from build123d import *

# Parameters (mm, degrees)
F1_DEPTH = 25.4
F3_DEPTH = 25.4
F4_DEPTH = 25.4


# Not quite as in the source:
# - a feature names something its author has since deleted; it is built from what else it names


with BuildPart() as f1:
    # F0 (on Top) → F1 (new body)
    with BuildSketch(Plane.XY):
        with BuildLine():
            ThreePointArc((128.3595710993, 553.8759422302), (1.1825358552, 549.8230168828), (-125.9080190212, 556.0210293531))
            Line((-125.9080190212, 556.0210293531), (-125.9080190212, -713.9789706469))
            ThreePointArc((-125.9080190212, -713.9789706469), (1.2643600135, -710.4779684085), (128.3595710993, -716.1240577698))
            Line((128.3595710993, -716.1240577698), (128.3595710993, 553.8759422302))
        make_face()
    extrude(amount=F1_DEPTH)

    # F2 (on face) → F3 (cut, through all)
    with BuildSketch(Plane.XY.offset(25.4)):
        with BuildLine():
            Line((21.1381499791, -78.9789706469), (0, -78.9789706469))
            Line((0, -78.9789706469), (0, -95.7576301918))
            ThreePointArc((0, -95.7576301918), (4.2283594629, -96.2864641581), (8.1962319091, -97.8403873742))
            Line((8.1962319091, -97.8403873742), (29.1618719602, -145.247048063))
            ThreePointArc((29.1618719602, -145.247048063), (59.1063769686, -142.7132397651), (62.4383196322, -112.8470092903))
            Line((62.4383196322, -112.8470092903), (27.7889794812, -88.7078500401))
            ThreePointArc((27.7889794812, -88.7078500401), (22.9597605864, -84.8714367544), (21.1381499791, -78.9789706469))
        make_face()
        with BuildLine():
            Line((0, -78.9789706469), (-21.1381499791, -78.9789706469))
            ThreePointArc((-21.1381499791, -78.9789706469), (-22.9597605864, -84.8714367544), (-27.7889794812, -88.7078500401))
            Line((-27.7889794812, -88.7078500401), (-62.4383196322, -112.8470092903))
            ThreePointArc((-62.4383196322, -112.8470092903), (-59.1063769686, -142.7132397651), (-29.1618719602, -145.247048063))
            Line((-29.1618719602, -145.247048063), (-8.3430390852, -97.9210786899))
            ThreePointArc((-8.3430390852, -97.9210786899), (-4.3094898358, -96.30729114), (0, -95.7576301918))
            Line((0, -95.7576301918), (0, -78.9789706469))
        make_face()
    extrude(amount=-F3_DEPTH, mode=Mode.SUBTRACT)

    # F2 (on face) → F4 (cut, through all)
    with BuildSketch(Plane.XY.offset(25.4)):
        with BuildLine():
            ThreePointArc((-27.7889794812, -69.2500912536), (-22.9597605864, -73.0865045393), (-21.1381499791, -78.9789706469))
            Line((-21.1381499791, -78.9789706469), (0, -78.9789706469))
            Line((0, -78.9789706469), (0, -62.2003111019))
            ThreePointArc((0, -62.2003111019), (-4.3094898358, -61.6506501538), (-8.3430390852, -60.0368626038))
            Line((-8.3430390852, -60.0368626038), (-29.1618719602, -12.7108932307))
            ThreePointArc((-29.1618719602, -12.7108932307), (-59.1063769686, -15.2447015287), (-62.4383196322, -45.1109320034))
            Line((-62.4383196322, -45.1109320034), (-27.7889794812, -69.2500912536))
        make_face()
        with BuildLine():
            Line((0, -62.2003111019), (0, -78.9789706469))
            Line((0, -78.9789706469), (21.1381499791, -78.9789706469))
            ThreePointArc((21.1381499791, -78.9789706469), (22.9597605864, -73.0865045393), (27.7889794812, -69.2500912536))
            Line((27.7889794812, -69.2500912536), (62.4383196322, -45.1109320034))
            ThreePointArc((62.4383196322, -45.1109320034), (59.1063769686, -15.2447015287), (29.1618719602, -12.7108932307))
            Line((29.1618719602, -12.7108932307), (8.1962319091, -60.1175539196))
            ThreePointArc((8.1962319091, -60.1175539196), (4.2283594629, -61.6714771356), (0, -62.2003111019))
        make_face()
    extrude(amount=-F4_DEPTH, mode=Mode.SUBTRACT)


solid = f1.part
Read the model definition and answer for the solid it produces. Units are mm, in the model's axes. A direction names the side the tool comes from. Round coordinates to 2 decimals unless told otherwise and drop trailing zeros. Order: outer loops, then holes, each group sorted by start corner. A loop starts at its lowest first (then second) coordinate and runs counter-clockwise, first axis right, second up. Notation, with made-up numbers: (41.5, -4) - (86.5, -4) arc R27 ccw to (86.5, 26) - close; hole circle Ø2 at (-29.5, 29.25). An arc over 180 degrees is marked (long way). Use one line per item in the form item = value. Start each with the question number.
(1) A flat-ended cylindrical pin translates along its axis: pin 1 Ø8 at (x, z) = (-59, 16) entering from +Y. Find the tip coordinate at first contact, or state that the pin passes through.
(2) Find the intervals of material crossed by line 1 along Y through (x, z) = (33.5, 14.25); line 2 along Y through (x, z) = (32, 1.25); line 3 along Y through (x, z) = (12, 10), in increasing order. Write a range as from..to.
(3) For faces 4 (the face through (-29, -71, 0)), 5 (the face through (44.87, -57.35, 12.88)), determine the directions among +Z, -Z, +X, -X, +Y, -Y from which every point of the face is accessible in a straight line to the end or side of a thin tool.
(4) The part is cut by section B-B (x = 50). Give the vertices of the cut face in (y, z).
(5) The part is cut by section A-A (z = 13.5). Give the vertices of the cut face in (x, y), then the cut area to 3 significant figures.
(6) Determine the mould class of faces 1 (the face through (-18.9, -121.92, 12.88)), 2 (the face through (-29, -71, 25.4)), 3 (the face through (2.96, 549.81, 12.52)) for opening direction Y: +Y half, -Y half, draft (parallel to the pull), parting line (faces both ways), or undercut.
Checked values:
q1.pin_1 = 551.67
q2.line_1 = -711.04..-147.61, -92.69..-65.27, -10.35..549.88
q2.line_2 = -711..-146.92, -91.64..-66.32, -11.03..549.86
q2.line_3 = -710.6..-106.44, -51.52..549.77
q3.face_4 = -Z, +X, -X, +Y, -Y
q3.face_5 = +Z, -Z
q4.outline = (-711.56, 0) - (-148.24, 0) - (-148.24, 25.4) - (-711.56, 25.4) - close; (-104.18, 0) - (-53.78, 0) - (-53.78, 25.4) - (-104.18, 25.4) - close; (-9.72, 0) - (550.17, 0) - (550.17, 25.4) - (-9.72, 25.4) - close
q5.outline = (-125.91, -713.98) arc R1769.36 cw to (128.36, -716.12) - (128.36, 553.88) arc R1579.35 cw to (-125.91, 556.02) - close; hole (-62.44, -112.85) arc R23.67 ccw to (-29.16, -145.25) - (-8.34, -97.92) arc R17.17 cw to (8.2, -97.84) - (29.16, -145.25) arc R23.67 ccw to (62.44, -112.85) - (27.79, -88.71) arc R10.44 cw to (27.79, -69.25) - (62.44, -45.11) arc R23.67 ccw to (29.16, -12.71) - (8.2, -60.12) arc R17.17 cw to (-8.34, -60.04) - (-29.16, -12.71) arc R23.67 ccw to (-62.44, -45.11) - (-27.79, -69.25) arc R10.44 cw to (-27.79, -88.71) - close
q5.area = 311,000 mm^2
q6.face_1 = undercut
q6.face_2 = draft
q6.face_3 = +Y half
